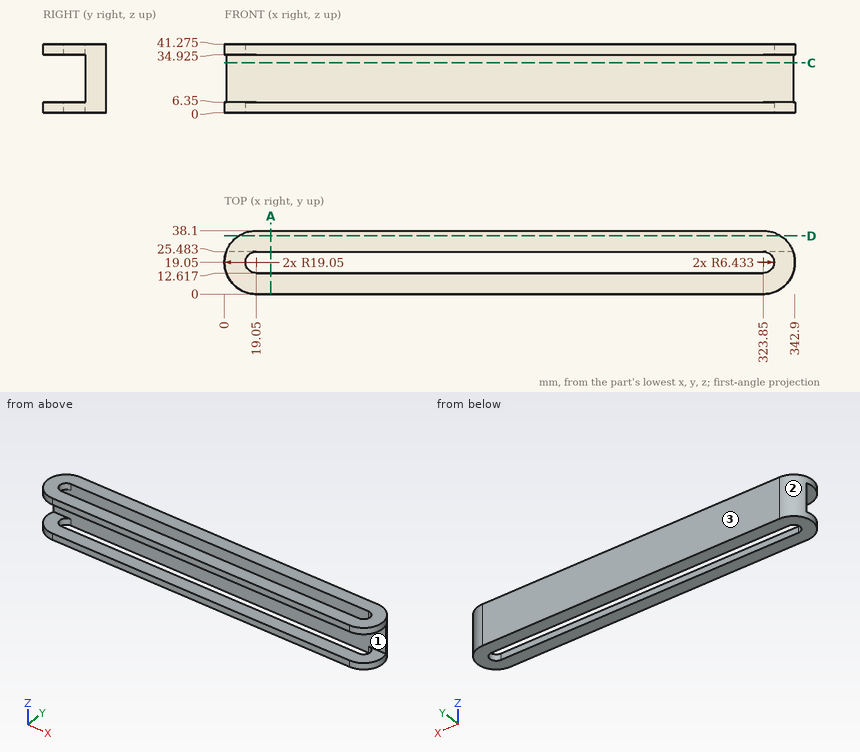
Answer from the drawing. Dimensions are ordinates in mm from the lowest x, y and z of the part. Round coordinates to 2 decimals unless told otherwise and drop trailing zeros. Write each loop counter-clockwise with the first axis right and the second up, starting at its lowest first coordinate (ties: lowest second). Pieces come first, ordered by that corner, then holes. Notation, with made-up numbers: M 86.5,53 L 111.5,53 A24 ccw 111.5,71 Z; hole C 88,70.5 d10. An arc over 180 degrees is marked long. Write each question's results on one line, items separated by ' | '. Start each with the question number.
Item 1: Find section D-D on y = 35. Write down the section's boundary in (x, z) (1 decimal).
Item 2: Find section A-A on x = 28. Give the number of separate pieces and of enclosed holes in the cut face, and give its area (3 significant figures).
Item 3: Given pin 1 Ø1 at (x, z) = (79, 9.5) entering from -Y; pin 2 Ø4 at (y, z) = (28, 13) entering from +X; pin 3 Ø1 at (x, y) = (143.5, 8) entering from -Z, each flat-ended and moving along its own axis, determine where each tip first touches the part or whether it passes through.
Item 4: Find section C-C on z = 30. Write down the section's boundary in (x, y).
Item 5: Straight lines are drawn through the part: probe 1 along X at (y, z) = (19, 39); probe 2 along Y at (x, z) = (36, 8); probe 3 along Y at (x, z) = (78, 40). For each, find the intervals that lie inside material, in ascending order.
Item 6: The mould has two halves that part along X. Classify the marked faces 1, 2 and 3: +X half, -X half, draft (parallel to the pull), parting line (faces both ways), or undercut.
Answer block:
1) outline: M 8.6,0 L 334.3,0 L 334.3,41.3 L 8.6,41.3 Z
2) separate pieces: 3 | enclosed holes: 0 | area: 681 mm²
3) pin 1: stops at y = 25.48 | pin 2: stops at x = 341.59 | pin 3: stops at z = 0
4) outline: M 1.12,25.48 L 341.78,25.48 A19.05 ccw 323.85,38.1 L 19.05,38.1 A19.05 ccw Z
5) probe 1: x = 0 to 12.62, 330.28 to 342.9 | probe 2: y = 25.48 to 38.1 | probe 3: y = 0 to 12.62, 25.48 to 38.1
6) face 1: undercut | face 2: -X half | face 3: draft
